```python
from build123d import *

# Parameters (mm, degrees)
F0_W     = 127
F0_H     = 254
F1_DEPTH = 2.54
F3_DEPTH = 25.4
F5_DEPTH = 25.4


with BuildPart() as f1:
    # F0 (on Front) → F1 (new body)
    with BuildSketch(Plane.XZ):
        with Locations((-91.982823, 130.963629)):
            Rectangle(F0_W, F0_H)
    extrude(amount=F1_DEPTH)

    # F2 (on face) → F3 (cut)
    with BuildSketch(Plane.XZ.offset(2.54)):
        with BuildLine():
            Line((-91.982823, 181.763629), (-91.982823, 232.563629))
            ThreePointArc((-91.982823, 232.563629), (-117.382823, 207.163629), (-91.982823, 181.763629))
        make_face()
        with BuildLine():
            ThreePointArc((-66.582823, 207.163629), (-74.02231, 225.124141), (-91.982823, 232.563629))
            Line((-91.982823, 232.563629), (-91.982823, 181.763629))
            ThreePointArc((-91.982823, 181.763629), (-74.02231, 189.203117), (-66.582823, 207.163629))
        make_face()
    extrude(amount=-F3_DEPTH, mode=Mode.SUBTRACT)

    # F4 (on face) → F5 (cut)
    with BuildSketch(Plane.XZ.offset(2.54)):
        with BuildLine():
            ThreePointArc((-91.982823, 80.163629), (-117.382823, 54.763629), (-91.982823, 29.363629))
            Line((-91.982823, 29.363629), (-91.982823, 80.163629))
        make_face()
        with BuildLine():
            Line((-91.982823, 80.163629), (-91.982823, 29.363629))
            ThreePointArc((-91.982823, 29.363629), (-74.02231, 36.803117), (-66.582823, 54.763629))
            ThreePointArc((-66.582823, 54.763629), (-74.02231, 72.724141), (-91.982823, 80.163629))
        make_face()
    extrude(amount=-F5_DEPTH, mode=Mode.SUBTRACT)


solid = f1.part
```
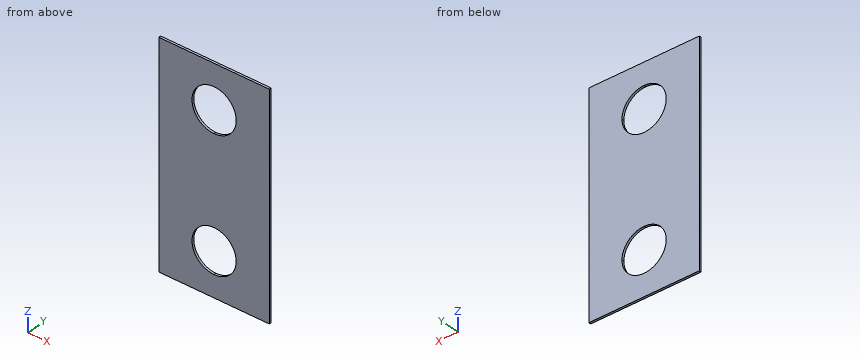
Model file for the job. Use its own axes, mm. Round coordinates to 2 decimals unless told otherwise and drop trailing zeros. Write each loop counter-clockwise with the first axis right and the second up, starting at its lowest first coordinate (ties: lowest second). Pieces come first, ordered by that corner, then holes. Notation, with made-up numbers: M 25.25,-33 L 60.25,-33 A18 cw 60.25,-12 Z; hole C 25,-4.75 d10. An arc over 180 degrees is marked long. Put each result on its own line as item: value.
Item 1: Probe L1, parallel to Z at x = -98, y = -0.75; L2, parallel to Z at x = -110, y = -2.05; L3, parallel to X at y = -0.9, z = 70. List the from-to ranges inside material, lowest first. Write a range as from..to.
Responses:
L1: 3.96..30.09, 79.44..182.49, 231.84..257.96
L2: 3.96..36.86, 72.67..189.26, 225.07..257.96
L3: -155.48..-112.31, -71.66..-28.48
Item 2: Cut at D-D (x = -79). List the corners of the cut face in (y, z).
Responses:
outline: M -2.54,3.96 L 0,3.96 L 0,32.93 L -2.54,32.93 Z; M -2.54,76.59 L 0,76.59 L 0,185.33 L -2.54,185.33 Z; M -2.54,228.99 L 0,228.99 L 0,257.96 L -2.54,257.96 Z
Item 3: Cut at A-A (y = -2.05). List the corners of the cut face in (x, z), and give its area (3 significant figures).
Responses:
outline: M -155.48,3.96 L -28.48,3.96 L -28.48,257.96 L -155.48,257.96 Z; hole M -91.98,29.36 A25.4 ccw -66.58,54.76 A25.4 ccw long Z; hole M -91.98,181.76 A25.4 ccw -66.58,207.16 A25.4 ccw long Z
area: 28,200 mm²
Item 4: Cut at B-B (x = -108.5). List the corners of the cut face in (y, z), and give its area (3 significant figures).
Responses:
outline: M -2.54,3.96 L 0,3.96 L 0,35.47 L -2.54,35.47 Z; M -2.54,74.06 L 0,74.06 L 0,187.87 L -2.54,187.87 Z; M -2.54,226.46 L 0,226.46 L 0,257.96 L -2.54,257.96 Z
area: 449 mm²
Item 5: Cut at C-C (z = 213). List the corners of the cut face in (x, y), and give its area (3 significant figures).
Responses:
outline: M -155.48,-2.54 L -116.7,-2.54 L -116.7,0 L -155.48,0 Z; M -67.26,-2.54 L -28.48,-2.54 L -28.48,0 L -67.26,0 Z
area: 197 mm²
